```python
from build123d import *

# Parameters (mm, degrees)
SKETCH1_R           = 1.5
BOSS_EXTRUDE1_DEPTH = 4


with BuildPart() as part:
    # Sketch1 → Boss-Extrude1 (new body)
    with BuildSketch(Plane(origin=(0, 0, 0), x_dir=(1, 0, 0), z_dir=(0, 1, 0))):
        Polygon((-75, -23), (-40, -23), (-40, -75), (40, -75), (40, -23), (75, -23), (75, 23), (40, 23), (40, 75), (-40, 75), (-40, 23), (-75, 23), align=None)
        with Locations(Location((20, 0, 0), (0, 0, 270))):
            Circle(SKETCH1_R, mode=Mode.SUBTRACT)
        with Locations(Location((65, 0, 0), (0, 0, 270))):
            Circle(SKETCH1_R, mode=Mode.SUBTRACT)
        with Locations(Location((-65, 0, 0), (0, 0, 90))):
            Circle(SKETCH1_R, mode=Mode.SUBTRACT)
        with Locations(Location((-20, 0, 0), (0, 0, 90))):
            Circle(SKETCH1_R, mode=Mode.SUBTRACT)
        with Locations(Location((-28, 63, 0), (0, 0, 270))):
            Circle(SKETCH1_R, mode=Mode.SUBTRACT)
        with Locations(Location((28, 63, 0), (0, 0, 270))):
            Circle(SKETCH1_R, mode=Mode.SUBTRACT)
        with Locations(Location((28, -63, 0), (0, 0, 270))):
            Circle(SKETCH1_R, mode=Mode.SUBTRACT)
        with Locations(Location((-28, -63, 0), (0, 0, 270))):
            Circle(SKETCH1_R, mode=Mode.SUBTRACT)
    extrude(amount=BOSS_EXTRUDE1_DEPTH)


solid = part.part
```
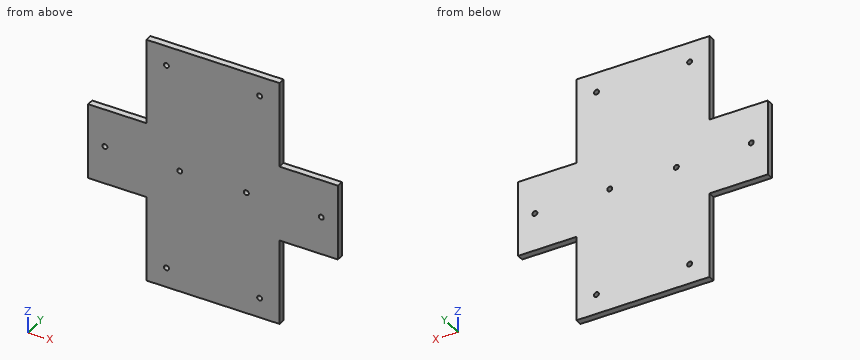
Here's how the part is built. I have some questions about the finished solid (model axes, mm). Coordinates: 2 decimals unless noted, no trailing zeros. Order: outer loops, then holes, each group sorted by start corner. A loop starts at its lowest first (then second) coordinate and runs counter-clockwise, first axis right, second up. Notation, with made-up numbers: (21.5, 19) - (46.5, 19) arc R27 ccw to (46.5, 49) - close; hole circle Ø11 at (-36.5, 82.5). An arc over 180 degrees is marked (long way). One line per question, with ' | ' between items.
(1) Will these pins go through, and if not, where does the flat tip stop? pin 1 (3.5 mm diameter, centred on x = 65, z = 0, fed in from +Y); pin 2 (1.2 mm diameter, centred on y = 3, z = 59, fed in from -X); pin 3 (1.2 mm diameter, centred on y = 1.5, z = 39, fed in from +X); pin 4 (1.2 mm diameter, centred on x = 61, y = 2.5, fed in from +Z).
Report:
pin 1: stops at y = 4 | pin 2: stops at x = -40 | pin 3: stops at x = 40 | pin 4: stops at z = 23
(2) Suppose I cut it at A-A on y = 1. State how many separate pieces and enclosed holes the cut face has, and give its area (3 significant figures).
Report:
separate pieces: 1 | enclosed holes: 8 | area: 15,200 mm2
(3) Suppose I cut it at C-C on z = -34.5. List the corners of the cut face in (x, y) for me, and give its area (3 significant figures).
Report:
outline: (-40, 0) - (40, 0) - (40, 4) - (-40, 4) - close | area: 320 mm2
(4) Suppose I cut it at B-B on x = -48. List the corners of the cut face in (y, z) for me.
Report:
outline: (0, -23) - (4, -23) - (4, 23) - (0, 23) - close
(5) If I drill on L1, parallel to X at y = 1.5, z = 0; L2, parallel to X at y = 1.95, z = 63; L3, parallel to Z at x = -20, y = 0.95, over which ranges is the centre line in solid material (lowest first)?
Report:
L1: x = -75 to -66.5, -63.5 to -21.5, -18.5 to 18.5, 21.5 to 63.5, 66.5 to 75 | L2: x = -40 to -29.5, -26.5 to 26.5, 29.5 to 40 | L3: z = -75 to -1.5, 1.5 to 75
